Answer from the drawing. Dimensions are ordinates in mm from the lowest x, y and z of the part. A direction names the side the tool comes from. Coordinates: 2 decimals unless noted, no trailing zeros. Order: outer loops, then holes, each group sorted by start corner. A loop starts at its lowest first (then second) coordinate and runs counter-clockwise, first axis right, second up. Notation, with made-up numbers: (23, -33) - (67, -33) arc R26 ccw to (67, -19) - close; hole circle Ø7 at (12.25, 13). An arc over 180 degrees is marked (long way). Answer as a JSON object with one key per item and string values. Group by question number.
1) A tool of negligible diameter and unlimited length cuts with its end or side. For the marked faces 1, 2 and 3, from which of +Z, -Z, +X, -X, +Y, -Y can it reach the whole face along a straight path? Write none if from no direction.
2) Section C-C (z = 27.5) is taken. Give the vertices of the cut face in (x, y), plus the area to 3 significant figures.
3) Find the intervals of material crossed by line 1 along Y through (x, z) = (45, 37); line 2 along X through (y, z) = (5.5, 71.5); line 3 along X through (y, z) = (10.25, 12), in increasing order.
4) Section B-B (y = 9) is taken. Give the vertices of the cut face in (x, z).
5) Section A-A (x = 45) is taken. Give the vertices of the cut face in (y, z).
6) Each of these flat-tipped pins is pushed along its axis until it touches: P1, Ø5.5, axis at x = 7.5, y = 10.5, coming from the -Z side; P2, Ø1.5, axis at x = 54, y = 14.5, coming from the +Z side; P3, Ø2, axis at x = 78, y = 9.5, coming from the +Z side; P4, Ø2.5, axis at x = 45, y = 9, coming from the -Z side. Where does it stop, or does it pass through?
7) Section D-D (y = 15) is taken. Give the vertices of the cut face in (x, z).
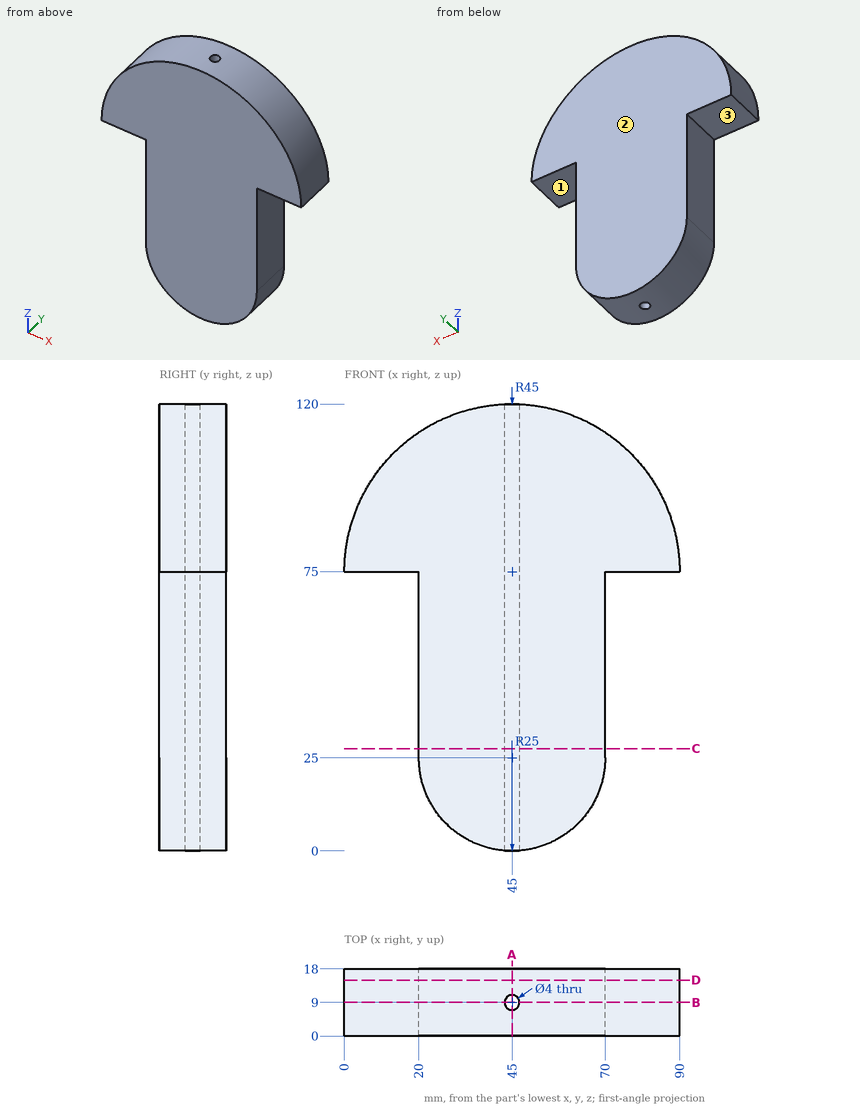
Report:
{
 "1": {"face 1": "-Z, +X, +Y, -Y", "face 2": "+Z, -Z, +X, -X, +Y", "face 3": "-Z, -X, +Y, -Y"},
 "2": {"outline": "(20, 0) - (70, 0) - (70, 18) - (20, 18) - close; hole circle Ø4 at (45, 9)", "area": "887 mm²"},
 "3": {"line 1": "y = 0 to 7, 11 to 18", "line 2": "x = 20 to 70", "line 3": "x = 23.65 to 43.44, 46.56 to 66.35"},
 "4": {"outline": "(0, 75) - (20, 75) - (20, 25) arc R25 ccw to (43, 0.08) - (43, 119.96) arc R45 ccw to start; (47, 0.08) arc R25 ccw to (70, 25) - (70, 75) - (90, 75) arc R45 ccw to (47, 119.96) - close"},
 "5": {"outline": "(0, 0) - (7, 0) - (7, 120) - (0, 120) - close; (11, 0) - (18, 0) - (18, 120) - (11, 120) - close"},
 "6": {"P1": "stops at z = 75", "P2": "stops at z = 119.24", "P3": "stops at z = 106.64", "P4": "passes through"},
 "7": {"outline": "(0, 75) - (20, 75) - (20, 25) arc R25 ccw to (70, 25) - (70, 75) - (90, 75) arc R45 ccw to start"}
}
